Here's how the part is built. I have some questions about the finished solid (model axes, mm). A direction names the side the tool comes from. Give positions to 0.01 mm unless a question says otherwise; leave off trailing zeros. Write each loop counter-clockwise with the first axis right and the second up, starting at its lowest first coordinate (ties: lowest second). Pieces come first, ordered by that corner, then holes. Notation, with made-up numbers: M -37.5,1 L -18.5,1 A22 cw -18.5,34 Z; hole C 62,-36 d3. An arc over 180 degrees is marked long. Answer as CSV lines item,"result". Start each with the question number.
Q1. Suppose I cut it at D-D (x = -34). Write out the boundary of the cut face in (y, z).
Q2. For pin 1 (12 mm diameter, centred on x = 1, z = 42, fed in from -Y), with a flat end and sliding along its axis, tell me the tip position at first contact or that it passes through.
Q3. Suppose I cut it at A-A (x = -10). Write out the boundary of the cut face in (y, z), then the cut area to 3 significant figures.
Q4. On a 3-axis mill with a long thin cutter (end or side, diameter ignored), from which of +Z, -Z, +X, -X, +Y, -Y can I reach the whole of each face in a straight line? I mean faces 4 (the flat face through (15, -4, 58)), 5 (the flat face through (-1, -5, 10)), 6 (the cylindrical face through (49, -9, 58)). Say none if no direction works.
Q5. Suppose I cut it at C-C (z = 30). Write out the boundary of the cut face in (x, y), then the cut area to 3 significant figures.
Q6. If I drill on line 1 along Z through (x, y) = (-45, -4); line 2 along X through (y, z) = (-8.75, 49); line 3 along X through (y, z) = (-1.75, 51.5), over which ranges is the centre line in solid material (lowest first)?
Q7. Suppose I cut it at B-B (y = -4.75). Write out the boundary of the cut face in (x, z), then the cut area to 3 significant figures.
Q8. Thinking about a two-plate mould opening in X: for faces 1 (the flat face through (-65, -5, 40)), 2 (the flat face through (-0.9, -10, 60.4)), 3 (the cylindrical face through (46.669, -4.056, 25.526)), which applies, +X half, -X half, draft (parallel to the pull), parting line (faces both ways), or undercut?
```python
from build123d import *

# Parameters (mm, degrees)
SKETCH022_W          = 130
SKETCH022_H          = 60
PAD008_DEPTH         = 10
SKETCH023_R          = 2.25
SKETCH023_R_2        = 1.75
SKETCH023_W          = 36
SKETCH023_H          = 36
POCKET014_DEPTH      = 10.001
POCKET014_DEPTH_BACK = 0.001
SKETCH024_W          = 100
SKETCH024_H          = 40
POCKET015_DEPTH      = 2
FILLET002_R          = 5


with BuildPart() as part:
    # Sketch022 → Pad008 (new body)
    with BuildSketch(Plane.XZ):
        with Locations((0, 40)):
            Rectangle(SKETCH022_W, SKETCH022_H)
    extrude(amount=PAD008_DEPTH)

    # Sketch023 (on Face6 of Pad008) → Pocket014 (cut, two sides)
    with BuildSketch(Plane.XZ.offset(10)) as pocket014_sk:
        with Locations((-25, 30)):
            Circle(SKETCH023_R)
        with Locations((-10, 30)):
            Circle(SKETCH023_R)
        with Locations((-45, 55)):
            Circle(SKETCH023_R_2)
        with Locations((-45, 25)):
            Circle(SKETCH023_R_2)
        with Locations((45, 55)):
            Circle(SKETCH023_R_2)
        with Locations((45, 25)):
            Circle(SKETCH023_R_2)
        with Locations((15, 40)):
            Rectangle(SKETCH023_W, SKETCH023_H)
    extrude(amount=-POCKET014_DEPTH, mode=Mode.SUBTRACT)
    extrude(pocket014_sk.sketch, amount=POCKET014_DEPTH_BACK, mode=Mode.SUBTRACT)

    # Sketch024 (on Face5 of Pocket014) → Pocket015 (cut)
    with BuildSketch(Plane.XZ.offset(10)):
        with Locations((0, 40)):
            Rectangle(SKETCH024_W, SKETCH024_H)
    extrude(amount=-POCKET015_DEPTH, mode=Mode.SUBTRACT)

    # Fillet002
    fillet002_edges = [part.edges().sort_by_distance(p)[0] for p in [
        (50, -9, 60),
        (50, -9, 20),
        (-50, -9, 20),
        (-50, -9, 60),
    ]]
    fillet(fillet002_edges, radius=FILLET002_R)


solid = part.part
```
Resolved:
1,outline,"M -10,10 L 0,10 L 0,70 L -10,70 L -10,60 L -8,60 L -8,20 L -10,20 Z"
2,pin 1,"y = -8"
3,outline,"M -10,10 L 0,10 L 0,27.75 L -8,27.75 L -8,20 L -10,20 Z; M -10,60 L -8,60 L -8,32.25 L 0,32.25 L 0,70 L -10,70 Z"
3,area,"484 mm^2"
4,face 4,"+Y, -Y"
4,face 5,"-Z, +X, -X, +Y, -Y"
4,face 6,"-Y"
5,outline,"M -65,-10 L -50,-10 L -50,-8 L -27.25,-8 L -27.25,0 L -65,0 Z; M -22.75,-8 L -12.25,-8 L -12.25,0 L -22.75,0 Z; M -7.75,-8 L -3,-8 L -3,0 L -7.75,0 Z; M 33,-8 L 50,-8 L 50,-10 L 65,-10 L 65,0 L 33,0 Z"
5,area,"740 mm^2"
6,line 1,"10 to 23.25, 26.75 to 53.25, 56.75 to 70"
6,line 2,"-65 to -50, 50 to 65"
6,line 3,"-65 to -3, 33 to 65"
7,outline,"M -65,10 L 65,10 L 65,70 L -65,70 Z; hole C -45,25 d3.5; hole C -45,55 d3.5; hole C -25,30 d4.5; hole C -10,30 d4.5; hole M -3,22 L 33,22 L 33,58 L -3,58 Z; hole C 45,25 d3.5; hole C 45,55 d3.5"
7,area,"6,430 mm^2"
8,face 1,"-X half"
8,face 2,"draft"
8,face 3,"undercut"
